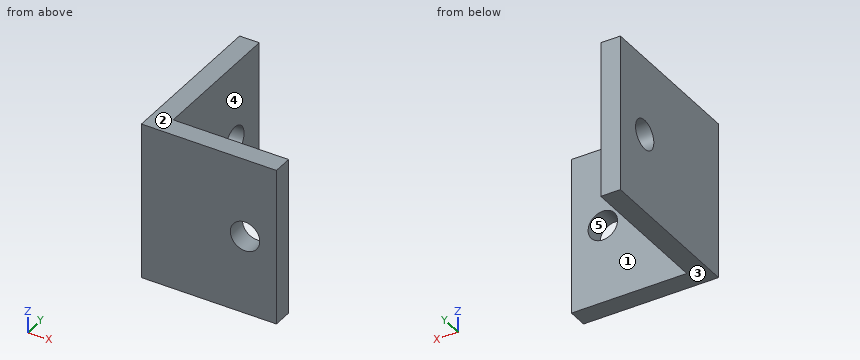
from build123d import *

# Parameters (mm, degrees)
BOSS_EXTRUDE1_DEPTH = 25.4
SKETCH2_R           = 2.38125
CUT_EXTRUDE1_DEPTH  = 41.642579606
SKETCH3_R           = 2.38125
CUT_EXTRUDE2_DEPTH  = 41.343844351


with BuildPart() as part:
    # Sketch1 → Boss-Extrude1 (new body)
    with BuildSketch(Plane.XY):
        Polygon((0, 0), (0, 25.654), (3.175, 25.654), (3.175, 3.175), (21.844, 3.175), (21.844, 0), align=None)
    extrude(amount=BOSS_EXTRUDE1_DEPTH)

    # Sketch2 → Cut-Extrude1 (cut, through all)
    with BuildSketch(Plane(origin=(3.175, 0, 0), x_dir=(0, 0, -1), z_dir=(1, 0, 0))):
        with Locations((-12.7, 19.304)):
            Circle(SKETCH2_R)
    extrude(amount=-CUT_EXTRUDE1_DEPTH, mode=Mode.SUBTRACT)

    # Sketch3 → Cut-Extrude2 (cut, through all)
    with BuildSketch(Plane(origin=(0, 3.175, 0), x_dir=(1, 0, 0), z_dir=(0, 1, 0))):
        with Locations(Location((16.764, -12.7, 0), (0, 0, 270))):
            Circle(SKETCH3_R)
    extrude(amount=-CUT_EXTRUDE2_DEPTH, mode=Mode.SUBTRACT)


solid = part.part
Can you work these out from the model? Positions are in its coordinate system, mm. Face numbers are marked on the shaded views. A direction names the side the tool comes from. Give positions to 0.01 mm unless a question says otherwise; leave off trailing zeros. Write each loop counter-clockwise with the first axis right and the second up, starting at its lowest first coordinate (ties: lowest second). Pieces come first, ordered by that corner, then holes. Notation, with made-up numbers: M 58,-13 L 103,-13 A17 ccw 103,-2 Z; hole C 43.25,62.25 d1. An arc over 180 degrees is marked long. Answer in a Markdown table with one row per item. Add a question column.
Item 1: On a 3-axis mill with a long thin cutter (end or side, diameter ignored), from which of +Z, -Z, +X, -X, +Y, -Y can I reach the whole of each face in a straight line? I mean the marked faces 1 and 2. Say none if no direction works.
Item 2: Imagine slicing it at A-A, the plane z = 12.7. Write out the boundary of the cut face in (x, y) (3 decimals).
Item 3: We'd pull the mould along Z, two halves only. Please class the marked faces 3, 4 and 5: released by +Z, released by -Z, zero draft, split by the parting line, or undercut.
Item 4: Imagine slicing it at D-D, the plane y = 10. Write out the boundary of the cut face in (x, z) (3 decimals), plus the area to 3 significant figures.
Item 5: Imagine slicing it at B-B, the plane x = 15.75. Write out the boundary of the cut face in (y, z) (3 decimals), plus the area to 3 significant figures.
Item 6: For pin 1 Ø5.5 at (y, z) = (19.304, 12.7) entering from +X (3 decimals); pin 2 Ø3 at (x, y) = (8.5, 6.5) entering from -Z; pin 3 Ø1.5 at (x, z) = (11.5, 4.5) entering from +Y (3 decimals), each with a flat end and sliding along its axis, tell me the tip position at first contact or that it passes through.
Item 7: Imagine slicing it at C-C, the plane z = 18. Write out the boundary of the cut face in (x, y) (3 decimals).
Item 8: Please list where these lines run through material, in increasing order: L1, parallel to Y at x = 1.5, z = 12.7; L2, parallel to X at y = 14, z = 14 (3 decimals).
Evaluation:
| question | item | result |
|---|---|---|
| 1 | face 1 | +Z, -Z, +X, +Y |
| 1 | face 2 | +Z, +X, -X, +Y, -Y |
| 2 | outline | M 0,0 L 14.383,0 L 14.383,3.175 L 3.175,3.175 L 3.175,16.923 L 0,16.923 Z; M 0,21.685 L 3.175,21.685 L 3.175,25.654 L 0,25.654 Z; M 19.145,0 L 21.844,0 L 21.844,3.175 L 19.145,3.175 Z |
| 3 | face 3 | released by -Z |
| 3 | face 4 | zero draft |
| 3 | face 5 | undercut |
| 4 | outline | M 0,0 L 3.175,0 L 3.175,25.4 L 0,25.4 Z |
| 4 | area | 80.6 mm² |
| 5 | outline | M 0,0 L 3.175,0 L 3.175,10.545 L 0,10.545 Z; M 0,14.855 L 3.175,14.855 L 3.175,25.4 L 0,25.4 Z |
| 5 | area | 67.0 mm² |
| 6 | pin 1 | stops at x = 3.175 |
| 6 | pin 2 | passes through |
| 6 | pin 3 | stops at y = 3.175 |
| 7 | outline | M 0,0 L 21.844,0 L 21.844,3.175 L 3.175,3.175 L 3.175,25.654 L 0,25.654 Z |
| 8 | L1 | y = 0 to 16.92, 21.69 to 25.65 |
| 8 | L2 | x = 0 to 3.175 |
